from build123d import *

# Parameters (mm, degrees)
SKETCH1_R           = 8
SKETCH1_R_2         = 3.5
BOSS_EXTRUDE1_DEPTH = 1.625
BOSS_EXTRUDE2_START = -0.75
SKETCH3_R           = 3.5
SKETCH3_R_2         = 2.5
BOSS_EXTRUDE2_DEPTH = 0.75
SKETCH4_R           = 3.5
SKETCH4_R_2         = 2.5
BOSS_EXTRUDE3_DEPTH = 0.5


with BuildPart() as part:
    # Sketch1 → Boss-Extrude1 (new, symmetric)
    with BuildSketch(Plane(origin=(0, 0, 0), x_dir=(1, 0, 0), z_dir=(0, 1, 0))):
        with Locations(Location((0, 0, 0), (0, 0, 90))):
            Circle(SKETCH1_R)
        with Locations(Location((0, 0, 0), (0, 0, 90))):
            Circle(SKETCH1_R_2, mode=Mode.SUBTRACT)
    extrude(amount=BOSS_EXTRUDE1_DEPTH, both=True)

    # Sketch2 → Cut-Revolve1 (revolve, cut)
    with BuildSketch(Plane(origin=(0, 0, 0), x_dir=(0, 0, -1), z_dir=(1, 0, 0)), mode=Mode.PRIVATE) as cut_revolve1_sk:
        with BuildLine():
            Line((-8, 0.75), (-8, -0.75))
            ThreePointArc((-8, -0.75), (-7.25, 0), (-8, 0.75))
        make_face()
    revolve(cut_revolve1_sk.sketch.rotate(Axis((0, 1.625, 0), (0, -1, 0)), 180), axis=Axis((0, 1.625, 0), (0, -1, 0)), mode=Mode.SUBTRACT)

    # Sketch3 → Boss-Extrude2 (add)
    with BuildSketch(Plane(origin=(0, 1.625, 0), x_dir=(1, 0, 0), z_dir=(0, 1, 0)).offset(BOSS_EXTRUDE2_START)):
        with Locations(Location((0, 0, 0), (0, 0, 90))):
            Circle(SKETCH3_R)
        with Locations(Location((0, 0, 0), (0, 0, 270))):
            Circle(SKETCH3_R_2, mode=Mode.SUBTRACT)
    extrude(amount=BOSS_EXTRUDE2_DEPTH)

    # Sketch4 → Boss-Extrude3 (add)
    with BuildSketch(Plane(origin=(0, 1.625, 0), x_dir=(1, 0, 0), z_dir=(0, 1, 0))):
        with Locations(Location((0, 0, 0), (0, 0, 90))):
            Circle(SKETCH4_R)
        with Locations(Location((0, 0, 0), (0, 0, 270))):
            Circle(SKETCH4_R_2, mode=Mode.SUBTRACT)
    extrude(amount=BOSS_EXTRUDE3_DEPTH)


solid = part.part
Geometry check sheet. Reference: the model listing, model coordinates, mm. A direction names the side the tool comes from. Round coordinates to 2 decimals unless told otherwise and drop trailing zeros. Order: outer loops, then holes, each group sorted by start corner. A loop starts at its lowest first (then second) coordinate and runs counter-clockwise, first axis right, second up. Notation, with made-up numbers: (-17.5, 56.25) - (30.5, 56.25) arc R31 cw to (30.5, 91.25) - close; hole circle Ø7 at (19, 62.5). An arc over 180 degrees is marked (long way). One line per question, with ' | ' between items. Start each with the question number.
(1) Release check for a two-part mould opening along Z. For faces 4 (the cylindrical face through (7.81, -1.18, 1.73)), 5 (the flat face through (2, 2.125, -2)), 6 (the cylindrical face through (-2.44, 1.49, -0.54)) record: released by +Z, released by -Z, zero draft, split by the parting line, or undercut.
(2) Depth check by flat-ended pin: pin 1 Ø2 at (y, z) = (-0.5, -4.5) entering from -X; pin 2 Ø2 at (x, y) = (1.5, 0) entering from -Z; pin 3 Ø1.5 at (x, z) = (-2.5, 4.5) entering from +Y (3 decimals). Enter the tip coordinate at first touch or a pass-through.
(3) Thickness scan on L1, parallel to Y at x = 3.75, z = -7 (3 decimals); L2, parallel to X at y = -0.9, z = 0; L3, parallel to X at y = 1.8, z = 0. Record the ranges inside material, lowest first. Write a range as [from, to].
(4) Sectioned sample at B-B on x = 0. Record the cut outline in (y, z) (3 decimals), and give its area (3 significant figures).
(5) Sectioned sample at A-A on z = 0. Record the cut outline in (x, y) (3 decimals), and give its area (3 significant figures).
(6) Sectioned sample at D-D on y = 1.15. Record the cut outline in (x, z).
(7) Access from +Z, -Z, +X, -X, +Y, -Y to the whole of each face (thin tool, end or side, straight path). Record for faces 1 (the cylindrical face through (7.81, 1.19, 1.73)), 2 (the flat face through (2, 0.875, -2)), 3 (the cylindrical face through (3.417, 1.872, 0.759)).
(8) Sectioned sample at C-C on y = -1.1. Record the cut outline in (x, z).
Conclusion:
1) face 4: split by the parting line | face 5: zero draft | face 6: undercut
2) pin 1: stops at x = -7.18 | pin 2: stops at z = -7.96 | pin 3: stops at y = 1.625
3) L1: y = [-1.625, -0.748], [0.748, 1.625] | L2: x = [-8, -3.5], [3.5, 8] | L3: x = [-3.5, -2.5], [2.5, 3.5]
4) outline: (-1.625, -8) - (-0.75, -8) arc R0.75 cw to (0.75, -8) - (1.625, -8) - (1.625, -3.5) - (2.125, -3.5) - (2.125, -2.5) - (0.875, -2.5) - (0.875, -3.5) - (-1.625, -3.5) - close; (-1.625, 3.5) - (0.875, 3.5) - (0.875, 2.5) - (2.125, 2.5) - (2.125, 3.5) - (1.625, 3.5) - (1.625, 8) - (0.75, 8) arc R0.75 cw to (-0.75, 8) - (-1.625, 8) - close | area: 30.0 mm2
5) outline: (-8, -1.625) - (-3.5, -1.625) - (-3.5, 0.875) - (-2.5, 0.875) - (-2.5, 2.125) - (-3.5, 2.125) - (-3.5, 1.625) - (-8, 1.625) - (-8, 0.75) arc R0.75 cw to (-8, -0.75) - close; (2.5, 0.875) - (3.5, 0.875) - (3.5, -1.625) - (8, -1.625) - (8, -0.75) arc R0.75 cw to (8, 0.75) - (8, 1.625) - (3.5, 1.625) - (3.5, 2.125) - (2.5, 2.125) - close | area: 30.0 mm2
6) outline: circle Ø16 at (0, 0); hole circle Ø5 at (0, 0)
7) face 1: +Y, -Y | face 2: -Y | face 3: +Y
8) outline: circle Ø16 at (0, 0); hole circle Ø7 at (0, 0)
